```python
from build123d import *

# Parameters (mm, degrees)
ESQUISSE1_R                  = 25
BOSS_EXTRU_1_DEPTH           = 113
ESQUISSE2_OUTSIDE_W          = 78.66
ESQUISSE2_OUTSIDE_H          = 78.66
ESQUISSE2_OUTSIDE_R          = 6
ENL_V_MAT_EXTRU_1_DEPTH      = 19
ESQUISSE3_OUTSIDE_W          = 78.66
ESQUISSE3_OUTSIDE_H          = 78.66
ESQUISSE3_OUTSIDE_R          = 6
ENL_V_MAT_EXTRU_3_DEPTH      = 89
ENL_V_MAT_EXTRU_3_DEPTH_BACK = 89
ESQUISSE4_OUTSIDE_W          = 78.66
ESQUISSE4_OUTSIDE_H          = 78.66
ESQUISSE4_OUTSIDE_R          = 2.5
ENL_V_MAT_EXTRU_4_DEPTH      = 36
ENL_V_MAT_EXTRU_4_DEPTH_BACK = 36
ESQUISSE8_R                  = 2
ENL_V_MAT_EXTRU_5_DEPTH      = 95
R_P_TITION_CIRCULAIRE2_COUNT = 4


with BuildPart() as part:
    # Esquisse1 → Boss.-Extru.1 (new body)
    with BuildSketch(Plane.XY):
        Circle(ESQUISSE1_R)
    extrude(amount=BOSS_EXTRU_1_DEPTH)

    # Esquisse2 outside → Enl_v. mat.-Extru.1 (cut)
    with BuildSketch(Plane.XY.offset(113)):
        Rectangle(ESQUISSE2_OUTSIDE_W, ESQUISSE2_OUTSIDE_H)
        Circle(ESQUISSE2_OUTSIDE_R, mode=Mode.SUBTRACT)
    extrude(amount=-ENL_V_MAT_EXTRU_1_DEPTH, mode=Mode.SUBTRACT)

    # Esquisse3 outside → Enl_v. mat.-Extru.3 (cut, two sides)
    with BuildSketch(Plane.XY) as enl_v_mat_extru_3_sk:
        Rectangle(ESQUISSE3_OUTSIDE_W, ESQUISSE3_OUTSIDE_H)
        Circle(ESQUISSE3_OUTSIDE_R, mode=Mode.SUBTRACT)
    extrude(amount=ENL_V_MAT_EXTRU_3_DEPTH, mode=Mode.SUBTRACT)
    extrude(enl_v_mat_extru_3_sk.sketch, amount=-ENL_V_MAT_EXTRU_3_DEPTH_BACK, mode=Mode.SUBTRACT)

    # Esquisse4 outside → Enl_v. mat.-Extru.4 (cut, two sides)
    with BuildSketch(Plane(origin=(0, 0, 0), x_dir=(-1, 0, 0), z_dir=(0, 0, -1))) as enl_v_mat_extru_4_sk:
        Rectangle(ESQUISSE4_OUTSIDE_W, ESQUISSE4_OUTSIDE_H)
        with Locations(Location((0, 0, 0), (0, 0, 180))):  # turned: the seam where the file's is
            Circle(ESQUISSE4_OUTSIDE_R, mode=Mode.SUBTRACT)
    extrude(amount=ENL_V_MAT_EXTRU_4_DEPTH, mode=Mode.SUBTRACT)
    extrude(enl_v_mat_extru_4_sk.sketch, amount=-ENL_V_MAT_EXTRU_4_DEPTH_BACK, mode=Mode.SUBTRACT)

    # Esquisse8 → Enl_v. mat.-Extru.5 (cut, through all)
    with BuildSketch(Plane.XY.offset(94)):
        with Locations((0, 20)):
            Circle(ESQUISSE8_R)
    enl_v_mat_extru_5 = extrude(amount=-ENL_V_MAT_EXTRU_5_DEPTH, mode=Mode.SUBTRACT)

    # R_p_tition circulaire2: Enl_v. mat.-Extru.5 ×4 about axis
    r_p_tition_circulaire2_axis = Axis((0, 0, 0), (0, 0, 1))
    for i in range(1, R_P_TITION_CIRCULAIRE2_COUNT):
        add(enl_v_mat_extru_5.rotate(r_p_tition_circulaire2_axis, i * 360 / R_P_TITION_CIRCULAIRE2_COUNT), mode=Mode.SUBTRACT)


solid = part.part
```
For this review, take the finished solid that the model builds, in its own axes (mm). A direction names the side the tool comes from. Round coordinates to 2 decimals unless told otherwise and drop trailing zeros. Write each loop counter-clockwise with the first axis right and the second up, starting at its lowest first coordinate (ties: lowest second). Pieces come first, ordered by that corner, then holes. Notation, with made-up numbers: (60.5, -39.5) - (90.5, -39.5) arc R13 ccw to (90.5, -27.5) - close; hole circle Ø4 at (5.5, 53). An arc over 180 degrees is marked (long way). Answer as CSV lines item,"result". Start each with the question number.
(1) Add section B-B, the plane x = -20. State the section outline as (y, z) points.
(2) Add section A-A, the plane y = 0. State the section outline as (x, z) points, plus the area to 3 significant figures.
(3) Mouldability with a two-part tool opening along Y and no side actions: class faces 4 (the cylindrical face through (23.846, 7.509, 91.465)), 5 (the flat face through (0, 0, 0)), 6 (the cylindrical face through (22, 0, 92)) as +Y half, -Y half, draft (parallel to the pull), parting line (faces both ways), or undercut.
(4) For line 1 (Y direction, x = 0, z = 92.75); line 2 (Z direction, x = -12.5, y = 5.5), list the stretches that pass through material, from the lowest coordinate up.
(5) For pin 1 (8 mm diameter, centred on y = -6, z = 50.5, fed in from +X); pin 2 (2.5 mm diameter, centred on x = -20, y = 0, fed in from -Z); pin 3 (5 mm diameter, centred on x = -4.5, y = -13, fed in from +Z); pin 4 (12 mm diameter, centred on x = -7, z = 50.5, fed in from -Y), all flat-tipped, find the tip position at first contact; note any pin that passes through.
(6) Machinability: for faces 1 (the cylindrical face through (0, -22, 92)), 2 (the flat face through (5, -5, 94)), 3 (the cylindrical face through (-2.5, -0.1, 17.7)), which of the approach directions +Z, -Z, +X, -X, +Y, -Y give a long, thin tool a straight path to every point of the face, cutting with its end or side? Answer none if there is none.
From the geometry:
1,outline,"(-15, 89) - (-2, 89) - (-2, 94) - (-15, 94) - close; (2, 89) - (15, 89) - (15, 94) - (2, 94) - close"
2,outline,"(-25, 89) - (-22, 89) - (-22, 94) - (-25, 94) - close; (-18, 89) - (-6, 89) - (-6, 36) - (-2.5, 36) - (-2.5, 0) - (2.5, 0) - (2.5, 36) - (6, 36) - (6, 89) - (18, 89) - (18, 94) - (6, 94) - (6, 113) - (-6, 113) - (-6, 94) - (-18, 94) - close; (22, 89) - (25, 89) - (25, 94) - (22, 94) - close"
2,area,"1,250 mm²"
3,face 4,"parting line"
3,face 5,"draft"
3,face 6,"undercut"
4,line 1,"y = -25 to -22, -18 to 18, 22 to 25"
4,line 2,"z = 89 to 94"
5,pin 1,"stops at x = 5.66"
5,pin 2,"passes through"
5,pin 3,"stops at z = 94"
5,pin 4,"stops at y = -5.92"
6,face 1,"+Z, -Z"
6,face 2,"+Z"
6,face 3,"-Z"
